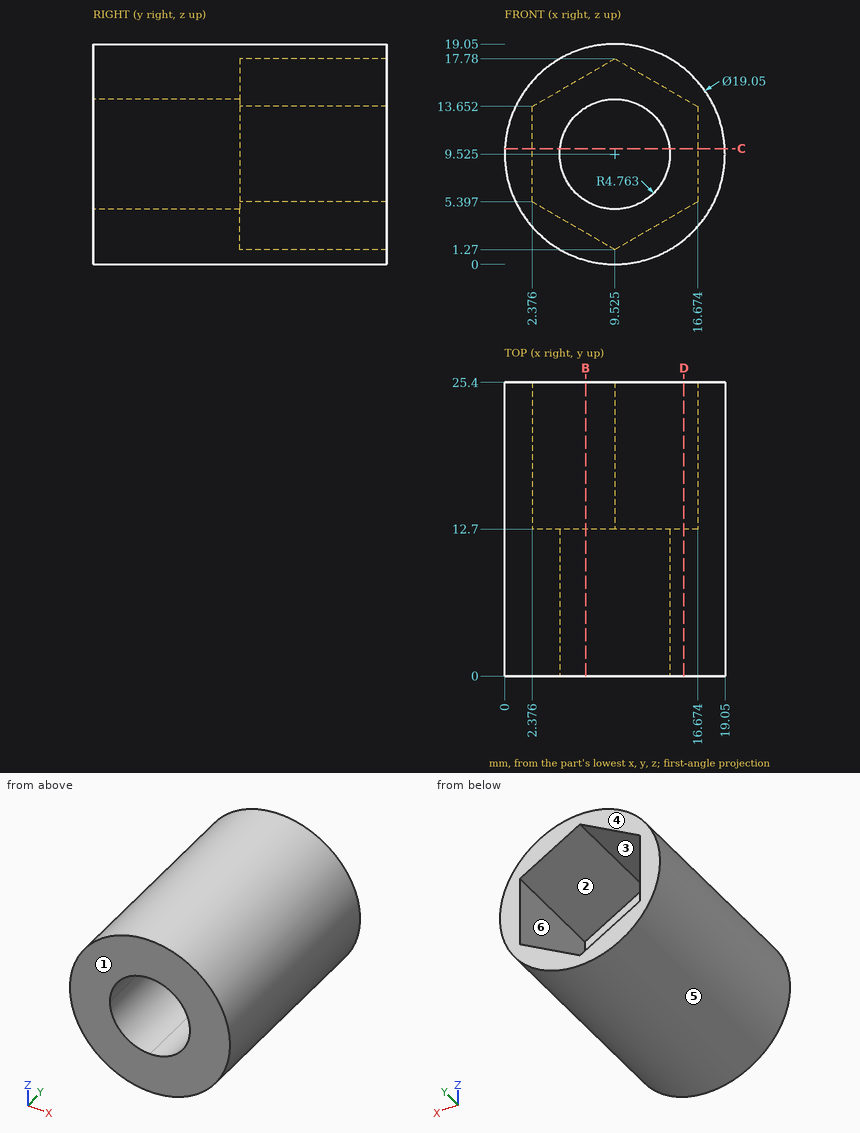
The drawing under review shows one solid part. Ordinate dimensions are in mm from its lowest x, y, z. A direction names the side the tool comes from. Round coordinates to 2 decimals unless told otherwise and drop trailing zeros. Loops run counter-clockwise (first coordinate to the right, second up) from the corner with the lowest first, then second, coordinate; pieces in that order, holes last. Notation, with made-up numbers: (39.5, 45.5) - (75.5, 45.5) arc R27 cw to (75.5, 82.5) - close; hole circle Ø9 at (-4, -30.5). An arc over 180 degrees is marked (long way). One line per question, with ' | ' between items.
Q1. For pin 1 (6 mm diameter, centred on x = 2.5, y = 11.5, fed in from -Z); pin 2 (2 mm diameter, centred on y = 12.5, z = 6, fed in from -X); pin 3 (3 mm diameter, centred on y = 21.5, z = 13, fed in from +X), all flat-tipped, find the tip position at first contact; note any pin that passes through.
Taken from the geometry:
pin 1: stops at z = 0.89 | pin 2: stops at x = 0.34 | pin 3: stops at x = 18.84
Q2. For line 1 along Y through (x, z) = (4, 14.25); line 2 along Z through (x, y) = (10.25, 12); line 3 along X through (y, z) = (17, 14) (1 decimal), list the stretches that pass through material, from the lowest coordinate up. Write a range as [from, to].
Taken from the geometry:
line 1: y = [0, 12.7] | line 2: z = [0.03, 4.82], [14.23, 19.02] | line 3: x = [1.1, 3], [16.1, 17.9]
Q3. Take a section at D-D (x = 15.5). Give the boundary of the cut face in (y, z), and give its area (3 significant figures).
Taken from the geometry:
outline: (0, 2.11) - (25.4, 2.11) - (25.4, 4.72) - (12.7, 4.72) - (12.7, 14.33) - (25.4, 14.33) - (25.4, 16.94) - (0, 16.94) - close | area: 255 mm²
Q4. Tool access review of the marked faces 1 and 2: name each direction out of +Z, -Z, +X, -X, +Y, -Y from which nothing blocks a thin tool from reaching the whole face with its end or side.
Taken from the geometry:
face 1: +Z, -Z, +X, -X, -Y | face 2: +Y
Q5. Take a section at C-C (z = 10). Give the boundary of the cut face in (x, y) (1 decimal).
Taken from the geometry:
outline: (0, 0) - (4.8, 0) - (4.8, 12.7) - (2.4, 12.7) - (2.4, 25.4) - (0, 25.4) - close; (14.3, 0) - (19, 0) - (19, 25.4) - (16.7, 25.4) - (16.7, 12.7) - (14.3, 12.7) - close
Q6. The part is to be moulded in two halves that separate along Z. For the marked faces 3, 4, 5 and 6, say which applies: released by +Z, released by -Z, zero draft, split by the parting line, or undercut.
Taken from the geometry:
face 3: undercut | face 4: zero draft | face 5: split by the parting line | face 6: undercut
Q7. Take a section at B-B (x = 7). Give the boundary of the cut face in (y, z).
Taken from the geometry:
outline: (0, 0.34) - (25.4, 0.34) - (25.4, 2.73) - (12.7, 2.73) - (12.7, 5.49) - (0, 5.49) - close; (0, 13.56) - (12.7, 13.56) - (12.7, 16.32) - (25.4, 16.32) - (25.4, 18.71) - (0, 18.71) - close
